Geometry: final body of the model. Coordinates: model frame, mm. A direction names the side the tool comes from. Give positions to 0.01 mm unless a question says otherwise; leave off trailing zeros. Write each loop counter-clockwise with the first axis right and the second up, starting at its lowest first coordinate (ties: lowest second). Pieces come first, ordered by that corner, then holes. Notation, with made-up numbers: (-21.75, 69) -> (20.25, 69) arc R23 ccw to (20.25, 86) -> close; hole circle Ø6 at (-29.5, 51.25). An arc over 180 degrees is marked (long way). Answer as a JSON object with one key per item and string values.
from build123d import *

# Parameters (mm, degrees)
SKETCH1_W                = 45
SKETCH1_H                = 16
SKETCH1_R                = 1.1
BOSS_EXTRUDE1_DEPTH      = 1.6
BOSS_EXTRUDE2_DEPTH      = 2
BOSS_EXTRUDE2_DEPTH_BACK = 6
SKETCH3_W                = 7
SKETCH3_H                = 16
BOSS_EXTRUDE3_DEPTH      = 10


with BuildPart() as part:
    # Sketch1 → Boss-Extrude1 (new body)
    with BuildSketch(Plane.XY):
        with Locations((22.5, 8)):
            Rectangle(SKETCH1_W, SKETCH1_H)
        with Locations((9, 14.25)):
            Circle(SKETCH1_R, mode=Mode.SUBTRACT)
        with Locations((9, 1.75)):
            Circle(SKETCH1_R, mode=Mode.SUBTRACT)
        with Locations((43.5, 14.25)):
            Circle(SKETCH1_R, mode=Mode.SUBTRACT)
        with Locations((43.5, 1.75)):
            Circle(SKETCH1_R, mode=Mode.SUBTRACT)
    extrude(amount=BOSS_EXTRUDE1_DEPTH)

    # Sketch2 → Boss-Extrude2 (add, two sides: drawn at the far end of the back side and taken through both)
    with BuildSketch(Plane(origin=(45, 0, 0), x_dir=(0, 0, -1), z_dir=(1, 0, 0)).offset(-BOSS_EXTRUDE2_DEPTH_BACK)):
        with BuildLine():
            Line((-1.6, 10.9), (-1.6, 5.1))
            ThreePointArc((-1.6, 5.1), (-3.2, 3.5), (-4.8, 5.1))
            Line((-4.8, 5.1), (-4.8, 10.9))
            ThreePointArc((-4.8, 10.9), (-3.2, 12.5), (-1.6, 10.9))
        make_face()
    extrude(amount=BOSS_EXTRUDE2_DEPTH + BOSS_EXTRUDE2_DEPTH_BACK)

    # Sketch3 → Boss-Extrude3 (add)
    with BuildSketch(Plane.XY.offset(1.6)):
        with Locations((3.5, 8)):
            Rectangle(SKETCH3_W, SKETCH3_H)
    extrude(amount=BOSS_EXTRUDE3_DEPTH)


solid = part.part
Q1. Cut plane D-D (y = 6). Return the cut outline in (x, z), and give its area (3 significant figures).
Values:
{"outline": "(0, 0) -> (45, 0) -> (45, 1.6) -> (47, 1.6) -> (47, 4.8) -> (39, 4.8) -> (39, 1.6) -> (7, 1.6) -> (7, 11.6) -> (0, 11.6) -> close", "area": "168 mm²"}
Q2. Cut plane C-C (z = 3.2). Return the cut outline in (x, y).
Values:
{"outline": "(0, 0) -> (7, 0) -> (7, 16) -> (0, 16) -> close; (39, 3.5) -> (47, 3.5) -> (47, 12.5) -> (39, 12.5) -> close"}
Q3. Cut plane B-B (x = 43.5). Return the cut outline in (y, z).
Values:
{"outline": "(0, 0) -> (0.65, 0) -> (0.65, 1.6) -> (0, 1.6) -> close; (2.85, 0) -> (13.15, 0) -> (13.15, 1.6) -> (10.9, 1.6) arc R1.6 ccw to (10.9, 4.8) -> (5.1, 4.8) arc R1.6 ccw to (5.1, 1.6) -> (2.85, 1.6) -> close; (15.35, 0) -> (16, 0) -> (16, 1.6) -> (15.35, 1.6) -> close"}
Q4. Set-up query: faces 5 (the flat face through (39, 8, 3)), 6 (the flat face through (3, 8, 11.6)), 7 (the flat face through (22, 8, 0)), 8 (the flat face through (45, 8, 1)), 9 (the flat face through (43, 8, 4.8)). Return all of +Z, -Z, +X, -X, +Y, -Y with unobstructed straight access to the full face (end or side cutting, diameter ignored); none if empty.
Values:
{"face 5": "+Z, +Y, -Y", "face 6": "+Z, +X, -X, +Y, -Y", "face 7": "-Z, +X, -X, +Y, -Y", "face 8": "-Z, +X, +Y, -Y", "face 9": "+Z, +X, +Y, -Y"}
Q5. First-contact query: P1, Ø1.6, axis at x = 46, y = 7, coming from the -Z side; P2, Ø2, axis at x = 9, y = 1.75, coming from the -Z side; P3, Ø5, axis at x = 24, y = 5.5, coming from the +Z side; P4, Ø1.7, axis at x = 45, y = 9.5, coming from the +Z side. Flat tips, straight axial feed; report the tip coordinate or a pass-through.
Values:
{"P1": "z = 1.6", "P2": "through", "P3": "z = 1.6", "P4": "z = 4.8"}
Q6. Material intervals for L1, parallel to Y at x = 43.5, z = 0.35; L2, parallel to X at y = 10.5, z = 3.75; L3, parallel to Z at x = 28, y = 14.5, sorted ascending. Write a range as from..to.
Values:
{"L1": "0..0.65, 2.85..13.15, 15.35..16", "L2": "0..7, 39..47", "L3": "0..1.6"}
Q7. Cut plane A-A (y = 1.75). Return the cut outline in (x, z).
Values:
{"outline": "(0, 0) -> (7.9, 0) -> (7.9, 1.6) -> (7, 1.6) -> (7, 11.6) -> (0, 11.6) -> close; (10.1, 0) -> (42.4, 0) -> (42.4, 1.6) -> (10.1, 1.6) -> close; (44.6, 0) -> (45, 0) -> (45, 1.6) -> (44.6, 1.6) -> close"}
Q8. Mould query, pull axis Y, two halves, no side actions, for faces 1 (the flat face through (7, 8, 7)), 2 (the cylindrical face through (44.55, 2.08, 0.79)), 3 (the flat face through (12, 16, 1)), 4 (the flat face through (12, 0, 1)). Classes: pulls with the +Y half, pulls with the -Y half, needs draft (parallel to the pull), parting line crosses it, or undercut.
Values:
{"face 1": "needs draft", "face 2": "undercut", "face 3": "pulls with the +Y half", "face 4": "pulls with the -Y half"}
